from build123d import *

# Parameters (mm, degrees)
ESTRUSIONE_ESTRUSIONE1_DEPTH   = 119
ESTRUSIONE_ESTRUSIONE1_2_DEPTH = 119
ESTRUSIONE_ESTRUSIONE2_DEPTH   = 2
ESTRUSIONE_ESTRUSIONE4_START   = -119
ESTRUSIONE_ESTRUSIONE4_DEPTH   = 2
RACCORDO1_R                    = 2
TAGLIO_ESTRUSIONE1_DEPTH       = 120.0000001
TAGLIO_ESTRUSIONE2_DEPTH       = 2
TAGLIO_ESTRUSIONE3_DEPTH       = 2
ESTRUSIONE_ESTRUSIONE5_DEPTH   = 10
ESTRUSIONE_ESTRUSIONE6_DEPTH   = 10


with BuildPart() as part:
    # Schizzo1 → Estrusione-Estrusione1 (new body)
    with BuildSketch(Plane.XY):
        with BuildLine():
            Line((-65.5, 80), (-63.5, 80))
            ThreePointArc((-63.5, 80), (-53.544927077, 45.865108989), (-26.801077658, 22.433062993))
            ThreePointArc((-26.801077658, 22.433062993), (-17.720444684, 15.202229716), (-12.936270867, 4.626099707))
            ThreePointArc((-12.936270867, 4.626099707), (-12.246718209, 3.459253333), (-10.971532063, 3))
            Line((-10.971532063, 3), (-10.5, 3))
            Line((-10.5, 3), (-10.5, 0))
            Line((-10.5, 0), (-12.5, 0))
            Line((-12.5, 0), (-12.5, -4))
            Line((-12.5, -4), (-14.5, -4))
            Line((-14.5, -4), (-14.5, 0))
            ThreePointArc((-14.5, 0), (-18.06581275, 12.226794372), (-27.645206088, 20.619931119))
            ThreePointArc((-27.645206088, 20.619931119), (-55.231381473, 44.789994311), (-65.5, 80))
        make_face()
    extrude(amount=ESTRUSIONE_ESTRUSIONE1_DEPTH)



with BuildPart() as body_2:
    # Schizzo1 → Estrusione-Estrusione1 2 (new body)
    with BuildSketch(Plane.XY):
        with BuildLine():
            Line((63.5, 80), (65.5, 80))
            ThreePointArc((65.5, 80), (55.231381473, 44.789994311), (27.645206088, 20.619931119))
            ThreePointArc((27.645206088, 20.619931119), (18.06581275, 12.226794372), (14.5, 0))
            Line((14.5, 0), (14.5, -4))
            Line((14.5, -4), (12.5, -4))
            Line((12.5, -4), (12.5, 0))
            Line((12.5, 0), (10.5, 0))
            Line((10.5, 0), (10.5, 3))
            Line((10.5, 3), (10.971532063, 3))
            ThreePointArc((10.971532063, 3), (12.246718209, 3.459253333), (12.936270867, 4.626099707))
            ThreePointArc((12.936270867, 4.626099707), (17.720444684, 15.202229716), (26.801077658, 22.433062993))
            ThreePointArc((26.801077658, 22.433062993), (53.544927077, 45.865108989), (63.5, 80))
        make_face()
    extrude(amount=ESTRUSIONE_ESTRUSIONE1_2_DEPTH)


with BuildPart() as part_1:
    add(part.part)

    add(body_2.part)  # Estrusione-Estrusione2 merges body 2
    # Schizzo2 → Estrusione-Estrusione2 (add)
    with BuildSketch(Plane.XY.offset(119)):
        with BuildLine():
            Line((65.5, 80), (-65.5, 80))
            ThreePointArc((-65.5, 80), (-55.231381473, 44.789994311), (-27.645206088, 20.619931119))
            ThreePointArc((-27.645206088, 20.619931119), (-18.06581275, 12.226794372), (-14.5, 0))
            Line((-14.5, 0), (-14.5, -4))
            Line((-14.5, -4), (14.5, -4))
            Line((14.5, -4), (14.5, 0))
            ThreePointArc((14.5, 0), (18.06581275, 12.226794372), (27.645206088, 20.619931119))
            ThreePointArc((27.645206088, 20.619931119), (55.231381473, 44.789994311), (65.5, 80))
        make_face()
    extrude(amount=-ESTRUSIONE_ESTRUSIONE2_DEPTH)

    # Schizzo2<4> → Estrusione-Estrusione4 (add)
    with BuildSketch(Plane.XY.offset(119).offset(ESTRUSIONE_ESTRUSIONE4_START)):
        with BuildLine():
            ThreePointArc((27.645206088, 20.619931119), (55.231381473, 44.789994311), (65.5, 80))
            Line((65.5, 80), (63.5, 80))
            ThreePointArc((63.5, 80), (53.544927077, 45.865108989), (26.801077658, 22.433062993))
            ThreePointArc((26.801077658, 22.433062993), (17.720444684, 15.202229716), (12.936270867, 4.626099707))
            ThreePointArc((12.936270867, 4.626099707), (12.246718209, 3.459253333), (10.971532063, 3))
            Line((10.971532063, 3), (10.5, 3))
            Line((10.5, 3), (10.5, 0))
            Line((10.5, 0), (12.5, 0))
            Line((12.5, 0), (12.5, -4))
            Line((12.5, -4), (14.5, -4))
            Line((14.5, -4), (14.5, 0))
            ThreePointArc((14.5, 0), (18.06581275, 12.226794372), (27.645206088, 20.619931119))
        make_face()
        with BuildLine():
            ThreePointArc((26.801077658, 22.433062993), (53.544927077, 45.865108989), (63.5, 80))
            Line((63.5, 80), (-63.5, 80))
            ThreePointArc((-63.5, 80), (-53.544927077, 45.865108989), (-26.801077658, 22.433062993))
            ThreePointArc((-26.801077658, 22.433062993), (-17.720444684, 15.202229716), (-12.936270867, 4.626099707))
            ThreePointArc((-12.936270867, 4.626099707), (-12.246718209, 3.459253333), (-10.971532063, 3))
            Line((-10.971532063, 3), (-10.5, 3))
            Line((-10.5, 3), (-10.5, 0))
            Line((-10.5, 0), (-12.5, 0))
            Line((-12.5, 0), (-12.5, -4))
            Line((-12.5, -4), (12.5, -4))
            Line((12.5, -4), (12.5, 0))
            Line((12.5, 0), (10.5, 0))
            Line((10.5, 0), (10.5, 3))
            Line((10.5, 3), (10.971532063, 3))
            ThreePointArc((10.971532063, 3), (12.246718209, 3.459253333), (12.936270867, 4.626099707))
            ThreePointArc((12.936270867, 4.626099707), (17.720444684, 15.202229716), (26.801077658, 22.433062993))
        make_face()
        with BuildLine():
            ThreePointArc((-26.801077658, 22.433062993), (-53.544927077, 45.865108989), (-63.5, 80))
            Line((-63.5, 80), (-65.5, 80))
            ThreePointArc((-65.5, 80), (-55.231381473, 44.789994311), (-27.645206088, 20.619931119))
            ThreePointArc((-27.645206088, 20.619931119), (-18.06581275, 12.226794372), (-14.5, 0))
            Line((-14.5, 0), (-14.5, -4))
            Line((-14.5, -4), (-12.5, -4))
            Line((-12.5, -4), (-12.5, 0))
            Line((-12.5, 0), (-10.5, 0))
            Line((-10.5, 0), (-10.5, 3))
            Line((-10.5, 3), (-10.971532063, 3))
            ThreePointArc((-10.971532063, 3), (-12.246718209, 3.459253333), (-12.936270867, 4.626099707))
            ThreePointArc((-12.936270867, 4.626099707), (-17.720444684, 15.202229716), (-26.801077658, 22.433062993))
        make_face()
    extrude(amount=ESTRUSIONE_ESTRUSIONE4_DEPTH)

    # Raccordo1
    raccordo1_edges = [part_1.edges().sort_by_distance(p)[0] for p in [
        (-14.5, -2, 0),
        (-18.06581275, 12.226794372, 0),
        (-55.231381473, 44.789994311, 0),
        (-55.231381473, 44.789994311, 119),
        (-18.06581275, 12.226794372, 119),
        (-14.5, -2, 119),
        (14.5, -2, 119),
        (55.231381473, 44.789994311, 119),
        (18.06581275, 12.226794372, 119),
        (55.231381473, 44.789994311, 0),
        (14.5, -2, 0),
        (18.06581275, 12.226794372, 0),
    ]]
    fillet(raccordo1_edges, radius=RACCORDO1_R)

    # Schizzo3 → Taglio-Estrusione1 (cut, through all)
    with BuildSketch(Plane.XY.offset(119)):
        with BuildLine():
            Line((-12.5, 0), (-12.5, -4))
            Line((-12.5, -4), (12.5, -4))
            Line((12.5, -4), (12.5, 0))
            Line((12.5, 0), (10.5, 0))
            Line((10.5, 0), (10.5, 3))
            Line((10.5, 3), (10.971532063, 3))
            ThreePointArc((10.971532063, 3), (11.534472979, 3.080860212), (12.051894373, 3.316902475))
            ThreePointArc((12.051894373, 3.316902475), (0, 12.5), (-12.051894373, 3.316902475))
            ThreePointArc((-12.051894373, 3.316902475), (-11.534472979, 3.080860212), (-10.971532063, 3))
            Line((-10.971532063, 3), (-10.5, 3))
            Line((-10.5, 3), (-10.5, 0))
            Line((-10.5, 0), (-12.5, 0))
        make_face()
    extrude(amount=-TAGLIO_ESTRUSIONE1_DEPTH, mode=Mode.SUBTRACT)

    # Schizzo5 → Taglio-Estrusione2 (cut)
    with BuildSketch(Plane.XY.offset(119)):
        with BuildLine():
            Line((-12.5, 0), (12.5, 0))
            ThreePointArc((12.5, 0), (0, 12.5), (-12.5, 0))
        make_face()
    extrude(amount=-TAGLIO_ESTRUSIONE2_DEPTH, mode=Mode.SUBTRACT)

    # Schizzo7 → Taglio-Estrusione3 (cut)
    with BuildSketch(Plane(origin=(0, 0, 0), x_dir=(-1, 0, 0), z_dir=(0, 0, -1))):
        with BuildLine():
            Line((12.5, 0), (-12.5, 0))
            ThreePointArc((-12.5, 0), (0, 12.5), (12.5, 0))
        make_face()
    extrude(amount=-TAGLIO_ESTRUSIONE3_DEPTH, mode=Mode.SUBTRACT)

    # Schizzo8 → Estrusione-Estrusione5 (add)
    with BuildSketch(Plane(origin=(0, 0, 0), x_dir=(-1, 0, 0), z_dir=(0, 0, -1))):
        with BuildLine():
            Line((-8.838834765, 8.838834765), (-10.606601718, 10.606601718))
            ThreePointArc((-10.606601718, 10.606601718), (0, 15), (10.606601718, 10.606601718))
            Line((10.606601718, 10.606601718), (8.838834765, 8.838834765))
            ThreePointArc((8.838834765, 8.838834765), (0, 12.5), (-8.838834765, 8.838834765))
        make_face()
    extrude(amount=ESTRUSIONE_ESTRUSIONE5_DEPTH)

    # Schizzo10 → Estrusione-Estrusione6 (add)
    with BuildSketch(Plane.XY.offset(119)):
        with BuildLine():
            Line((8.838834765, 8.838834765), (10.606601718, 10.606601718))
            ThreePointArc((10.606601718, 10.606601718), (0, 15), (-10.606601718, 10.606601718))
            Line((-10.606601718, 10.606601718), (-8.838834765, 8.838834765))
            ThreePointArc((-8.838834765, 8.838834765), (0, 12.5), (8.838834765, 8.838834765))
        make_face()
    extrude(amount=ESTRUSIONE_ESTRUSIONE6_DEPTH)


solid = part_1.part
Design review of the part built by this model. Coordinates are the model's own, in mm. A direction names the side the tool comes from. Give positions to 0.01 mm unless a question says otherwise; leave off trailing zeros. Write each loop counter-clockwise with the first axis right and the second up, starting at its lowest first coordinate (ties: lowest second). Pieces come first, ordered by that corner, then holes. Notation, with made-up numbers: M 18,61.25 L 62,61.25 A7 ccw 62,65.25 Z; hole C 89.25,67 d8. An arc over 180 degrees is marked long. Answer as a JSON object with one key per item and string values. Group by question number.
1) Clearance check with flat-ended pins moving along their axes: pin 1 Ø1 at (x, y) = (-11.5, 1.5) entering from -Z; pin 2 Ø1.6 at (x, y) = (11, 1.5) entering from +Z; pin 3 Ø0.5 at (x, z) = (11, 57.5) entering from +Y. State where each tip first meets the part, or that it passes through.
2) Tool access review of faces 5 (the face through (14.5, -2, 59)), 6 (the face through (12.5, -2, 60)), 7 (the face through (-14.5, -2, 59)), 8 (the face through (-1, 51, 117)): name each direction out of +Z, -Z, +X, -X, +Y, -Y from which nothing blocks a thin tool from reaching the whole face with its end or side.
3) We need section B-B (x = -5.5). Give the boundary of the cut face in (y, z).
4) For line 1 along Z through (x, y) = (-50.5, 51.5); line 2 along X through (y, z) = (1, 40.5); line 3 along X through (y, z) = (64, 49.5), list the stretches that pass through material, from the lowest coordinate up.
5) Mouldability with a two-part tool opening along X and no side actions: class faces 1 (the face through (-17.969, 12.074, 58.695)), 2 (the face through (53.27, 45.44, 58.7)), 3 (the face through (18.164, 12.379, 58.695)), 4 (the face through (0, 15, 124)) as released by +X, released by -X, zero draft, split by the parting line, or undercut.
6) We need section A-A (z = 8). Give the boundary of the cut face in (x, y), and give its area (3 significant figures).
Answer key:
{
 "1": {"pin 1": "stops at z = 2", "pin 2": "stops at z = 117", "pin 3": "stops at y = 3.02"},
 "2": {"face 5": "+Z, -Z, +X, -Y", "face 6": "+Z, -Z, -Y", "face 7": "+Z, -Z, -X, -Y", "face 8": "+Y"},
 "3": {"outline": "M 11.22,-10 L 13.96,-10 L 13.96,0 L 80,0 L 80,2 L 11.22,2 Z; M 11.22,117 L 80,117 L 80,119 L 13.96,119 L 13.96,129 L 11.22,129 Z"},
 "4": {"line 1": "z = 0 to 2, 117 to 119", "line 2": "x = -14.52 to -10.5, 10.5 to 14.52", "line 3": "x = -63.52 to -61.45, 61.45 to 63.52"},
 "5": {"face 1": "released by -X", "face 2": "undercut", "face 3": "released by +X", "face 4": "split by the parting line"},
 "6": {"outline": "M -65.5,80 A65.5 ccw -27.65,20.62 A22.75 cw -14.5,0 L -14.5,-4 L -12.5,-4 L -12.5,0 L -10.5,0 L -10.5,3 L -10.97,3 A2 cw -12.94,4.63 A24.75 ccw -26.8,22.43 A63.5 cw -63.5,80 Z; M 10.5,0 L 12.5,0 L 12.5,-4 L 14.5,-4 L 14.5,0 A22.75 cw 27.65,20.62 A65.5 ccw 65.5,80 L 63.5,80 A63.5 cw 26.8,22.43 A24.75 ccw 12.94,4.63 A2 cw 10.97,3 L 10.5,3 Z", "area": "430 mm²"}
}
